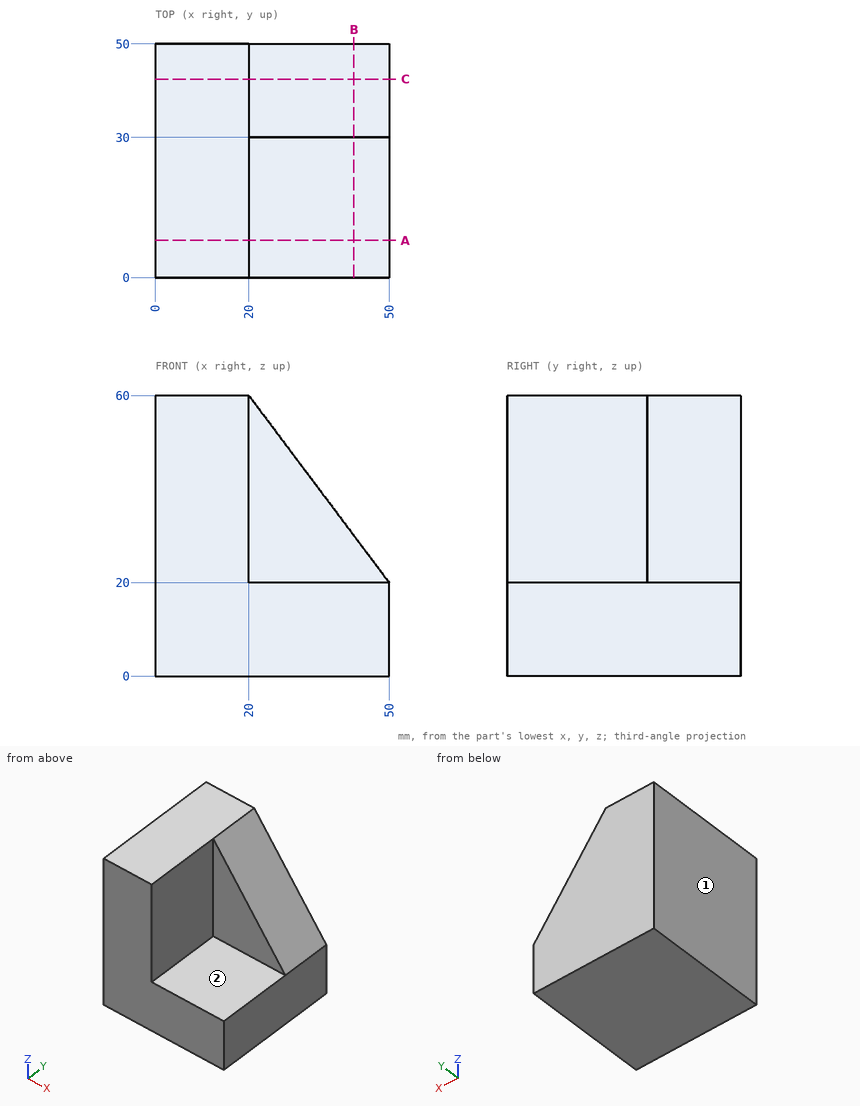
Geometry: see drawing. Coordinates: mm, zero at the bounding-box minimum. A direction names the side the tool comes from. Coordinates: 2 decimals unless noted, no trailing zeros. Loops run counter-clockwise (first coordinate to the right, second up) from the corner with the lowest first, then second, coordinate; pieces in that order, holes last. Notation, with made-up numbers: M -12,17.5 L 25,17.5 A26 cw 25,42.5 Z; hole C -1.75,81 d1. An arc over 180 degrees is marked long. Put each result on its own line as item: value. Start each with the question number.
1) Cut plane C-C on y = 42.5. Return the cut outline in (x, z).
2) Cut plane B-B on x = 42.5. Return the cut outline in (y, z), then the cut area to 3 significant figures.
3) Contact query for flat-ended pins moving along their axis: pin 1 Ø9 at (x, z) = (36.5, 30) entering from -Y; pin 2 Ø12 at (y, z) = (19.5, 34.5) entering from +X. Output: stop coordinate, or through.
4) Reachability of the marked faces 1 and 2 from +Z, -Z, +X, -X, +Y, -Y: full face, straight path, thin tool, end or side. Return the list, or none.
5) Ray query, L1, parallel to X at y = 7, z = 54.5; L2, parallel to Y at x = 24, z = 43. Return the intervals inside material, ascending. Write a range as from..to.
6) Cut plane A-A on y = 8. Return the cut outline in (x, z), then the cut area to 3 significant figures.
The answers:
1. outline: M 0,0 L 50,0 L 50,20 L 20,60 L 0,60 Z
2. outline: M 0,0 L 50,0 L 50,30 L 30,30 L 30,20 L 0,20 Z
2. area: 1,200 mm²
3. pin 1: stops at y = 30
3. pin 2: stops at x = 20
4. face 1: +Z, -Z, -X, +Y, -Y
4. face 2: +Z, +X, -Y
5. L1: x = 0..20
5. L2: y = 30..50
6. outline: M 0,0 L 50,0 L 50,20 L 20,20 L 20,60 L 0,60 Z
6. area: 1,800 mm²
